```python
from build123d import *

# Parameters (mm, degrees)
ESBO_O2_R                  = 4.5
RESSALTO_EXTRUS_O1_DEPTH   = 60
CORTE_EXTRUS_O1_DEPTH      = 86.164546614
CORTE_EXTRUS_O6_DEPTH      = 79.549347547
CORTE_EXTRUS_O6_DEPTH_BACK = 79.549347547
CORTE_EXTRUS_O7_DEPTH      = 79.549347547
CORTE_EXTRUS_O7_DEPTH_BACK = 79.549347547
FILETE1_R                  = 2


with BuildPart() as part:
    # Esboço2 → Ressalto-extrusão1 (new body)
    with BuildSketch(Plane(origin=(0, 0, 0), x_dir=(1, 0, 0), z_dir=(0, 1, 0))):
        with BuildLine():
            Line((38, 19), (-38, 19))
            Line((-38, 19), (-38, 9))
            ThreePointArc((-38, 9), (-47, 0), (-38, -9))
            Line((-38, -9), (-38, -19))
            Line((-38, -19), (38, -19))
            Line((38, -19), (38, -9))
            ThreePointArc((38, -9), (47, 0), (38, 9))
            Line((38, 9), (38, 19))
        make_face()
        with Locations(Location((-38, 0, 0), (0, 0, 270))):
            Circle(ESBO_O2_R, mode=Mode.SUBTRACT)
        with Locations(Location((38, 0, 0), (0, 0, 270))):
            Circle(ESBO_O2_R, mode=Mode.SUBTRACT)
    extrude(amount=RESSALTO_EXTRUS_O1_DEPTH)

    # Esboço3 → Corte-extrusão1 (cut, through all)
    with BuildSketch(Plane.XY.offset(19)):
        with BuildLine():
            Line((13.5, 60), (-13.5, 60))
            ThreePointArc((-13.5, 60), (0, 46.5), (13.5, 60))
        make_face()
    extrude(amount=-CORTE_EXTRUS_O1_DEPTH, mode=Mode.SUBTRACT)

    # Esboço4 → Corte-extrusão6 (cut, two sides: drawn at the far end of the back side and taken through both)
    with BuildSketch(Plane.XY.offset(-CORTE_EXTRUS_O6_DEPTH_BACK)):
        Polygon((-214.350715587, 153.88057247), (-47, 20), (-22, 0), (145.350715587, -133.88057247), (-122.410429352, -468.582003645), (-482.111860527, -180.820858705), align=None)
    extrude(amount=CORTE_EXTRUS_O6_DEPTH + CORTE_EXTRUS_O6_DEPTH_BACK, mode=Mode.SUBTRACT)

    # Esboço5 → Corte-extrusão7 (cut, two sides: drawn at the far end of the back side and taken through both)
    with BuildSketch(Plane.XY.offset(-CORTE_EXTRUS_O7_DEPTH_BACK)):
        Polygon((214.350715587, 153.88057247), (47, 20), (22, 0), (-145.350715587, -133.88057247), (122.410429352, -468.582003645), (482.111860527, -180.820858705), align=None)
    extrude(amount=CORTE_EXTRUS_O7_DEPTH + CORTE_EXTRUS_O7_DEPTH_BACK, mode=Mode.SUBTRACT)

    # Filete1
    filete1_edges = [part.edges().sort_by_distance(p)[0] for p in [
        (-38, 36.4, -19),
        (38, 36.4, -19),
        (38, 36.4, 19),
        (-38, 36.4, 19),
        (0, 0, -19),
        (0, 0, 19),
        (-30, 6.4, -19),
        (-30, 6.4, 19),
        (-22, 0, 0),
        (30, 6.4, 19),
        (22, 0, 0),
        (30, 6.4, -19),
    ]]
    fillet(filete1_edges, radius=FILETE1_R)


solid = part.part
```
For this review, take the finished solid that the model builds, in its own axes (mm). A direction names the side the tool comes from. Give positions to 0.01 mm unless a question says otherwise; leave off trailing zeros. Write each loop counter-clockwise with the first axis right and the second up, starting at its lowest first coordinate (ties: lowest second). Pieces come first, ordered by that corner, then holes. Notation, with made-up numbers: M -1,64.25 L 22,64.25 A22 cw 22,90.25 Z; hole C 23,63.5 d5. An arc over 180 degrees is marked long. Answer as a JSON object with one key per item and string values. Group by question number.
Item 1: For pin 1 Ø4 at (y, z) = (38.5, -15) entering from -X; pin 2 Ø1 at (x, z) = (-6.5, -14.5) entering from +Y; pin 3 Ø4 at (y, z) = (32, 13.5) entering from +X; pin 4 Ø7 at (x, z) = (38, 0) entering from +Y, all flat-tipped, find the tip position at first contact; note any pin that passes through.
Item 2: Tool access review of faces 1 (the flat face through (-38, 36, -13)), 2 (the cylindrical face through (37.4, 36.73, -18.43)), 3 (the flat face through (38, 36, 13)): name each direction out of +Z, -Z, +X, -X, +Y, -Y from which nothing blocks a thin tool from reaching the whole face with its end or side.
Item 3: Consider section C-C on z = 15. Write out the cut boundary in (x, y).
Item 4: Consider section D-D on y = 51. Write out the cut boundary in (x, z), plus the area to 3 significant figures.
Item 5: Draft analysis for pull direction X (two halves, no side actions). For faces 4 (the cylindrical face through (37.4, 36.73, 18.43)), 5 (the cylindrical face through (-29.81, 6.98, 18.4)), 6 (the cylindrical face through (-0.297, 46.503, 0.266)), state which applies: +X half, -X half, draft (parallel to the pull), parting line (faces both ways), or undercut.
Item 6: Consider section B-B on y = 33. Write out the cut boundary in (x, z), plus the area to 3 significant figures.
Item 7: Consider section A-A on z = 0. Write out the cut boundary in (x, y).
Item 8: For probe 1 along X at (y, z) = (29, 0); probe 2 along X at (y, z) = (32.5, 14); probe 3 along X at (y, z) = (52.5, -16), list the stretches that pass through material, from the lowest coordinate up. Write a range as [from, to].
Check result:
{
 "1": {"pin 1": "stops at x = -38", "pin 2": "stops at y = 48.46", "pin 3": "stops at x = 38", "pin 4": "passes through"},
 "2": {"face 1": "-Z, -X, +Y, -Y", "face 2": "-Z, +X, +Y, -Y", "face 3": "+Z, +X, +Y, -Y"},
 "3": {"outline": "M -38,12.8 L -22.55,0.44 A2 ccw -21.3,0 L 21.3,0 A2 ccw 22.55,0.44 L 38,12.8 L 38,60 L 13.5,60 A13.5 cw -13.5,60 L -38,60 Z"},
 "4": {"outline": "M -38,-17 A2 ccw -36,-19 L -10.06,-19 L -10.06,19 L -36,19 A2 ccw -38,17 L -38,9 A9 ccw -38,-9 Z; M 10.06,-19 L 36,-19 A2 ccw 38,-17 L 38,-9 A9 ccw 38,9 L 38,17 A2 ccw 36,19 L 10.06,19 Z; hole C -38,0 d9; hole C 38,0 d9", "area": "2,250 mm^2"},
 "5": {"face 4": "+X half", "face 5": "-X half", "face 6": "undercut"},
 "6": {"outline": "M -38,-17 A2 ccw -36,-19 L 36,-19 A2 ccw 38,-17 L 38,-9 A9 ccw 38,9 L 38,17 A2 ccw 36,19 L -36,19 A2 ccw -38,17 L -38,9 A9 ccw -38,-9 Z; hole C -38,0 d9; hole C 38,0 d9", "area": "3,010 mm^2"},
 "7": {"outline": "M -47,20 L -42.5,16.4 L -42.5,60 L -47,60 Z; M -33.5,9.2 L -22.55,0.44 A2 ccw -21.3,0 L 21.3,0 A2 ccw 22.55,0.44 L 33.5,9.2 L 33.5,60 L 13.5,60 A13.5 cw -13.5,60 L -33.5,60 Z; M 42.5,16.4 L 47,20 L 47,60 L 42.5,60 Z"},
 "8": {"probe 1": "x = [-47, -42.5], [-33.5, 33.5], [42.5, 47]", "probe 2": "x = [-38, 38]", "probe 3": "x = [-38, -11.22], [11.22, 38]"}
}
